Autodesk Inventor part; units mm, degrees
ref_plane "YZ Plane" through (0, 0, 0) normal (1, 0, 0) x (0, 1, 0)
ref_plane "XZ Plane" through (0, 0, 0) normal (0, 1, 0) x (-1, 0, 0)
ref_plane "XY Plane" through (0, 0, 0) normal (0, 0, 1) x (1, 0, 0)
sketch "Sketch1" plane through (0, 0, 0) normal (0, 0, 1) x (1, 0, 0)
  line L0 (7, 20) -> (20, 20)
  line L1 (0, 13) -> (0, 0)
  arc A0 (7, 20) -> (0, 13) centre (7, 13) ccw
  dimension "d3" = 7
  dimension "d10" = 20
  dimension "d11" = 20
sketch "Sketch2" plane through (0, 0, 0) normal (0, 1, 0) x (-1, 0, 0)
  circle A0 centre (0, 0) radius 0.4
  circle A1 centre (0, 0) radius 0.3
  dimension "d6" = 0.8
  dimension "d9" = 0.6
sweep "Sweep1" add profiles "Sketch2" path "Sketch1"
properties part number "TorsionOscillator-FillLine-Coupling" material "Nickel-Copper Alloy 400"
Could you check a few things on this model? Use its own coordinates, in mm. Round coordinates to 2 decimals unless told otherwise and drop trailing zeros. Write each loop counter-clockwise with the first axis right and the second up, starting at its lowest first coordinate (ties: lowest second). Pieces come first, ordered by that corner, then holes.
(1) If I drill on probe 1 along Y at (x, z) = (1.5, 0.15), over which ranges is the centre line in solid material (lowest first)?
Findings below:
probe 1: y = 16.7 to 16.9, 17.74 to 17.91
(2) Suppose I cut it at B-B on x = 9.5. Write out the boundary of the cut face in (y, z).
Findings below:
outline: circle Ø0.8 at (20, 0); hole circle Ø0.6 at (20, 0)
(3) For pin 1 (12 mm diameter, centred on x = 13, y = 8, fed in from +Z), with a flat end and sliding along its axis, tell me the tip position at first contact or that it passes through.
Findings below:
pin 1: passes through
(4) Suppose I cut it at A-A on z = 0. Write out the boundary of the cut face in (x, y), and give its area (3 significant figures).
Findings below:
outline: (-0.4, 0) - (-0.3, 0) - (-0.3, 13) arc R7.3 cw to (7, 20.3) - (20, 20.3) - (20, 20.4) - (7, 20.4) arc R7.4 ccw to (-0.4, 13) - close; (0.3, 0) - (0.4, 0) - (0.4, 13) arc R6.6 cw to (7, 19.6) - (20, 19.6) - (20, 19.7) - (7, 19.7) arc R6.7 ccw to (0.3, 13) - close
area: 7.40 mm2
(5) Suppose I cut it at C-C on y = 9.25. Write out the boundary of the cut face in (x, z).
Findings below:
outline: circle Ø0.8 at (0, 0); hole circle Ø0.6 at (0, 0)
